Design review of the part built by this model. Coordinates are the model's own, in mm. A direction names the side the tool comes from. Round coordinates to 2 decimals unless told otherwise and drop trailing zeros. Loops run counter-clockwise (first coordinate to the right, second up) from the corner with the lowest first, then second, coordinate; pieces in that order, holes last. Notation, with made-up numbers: (-32.5, 52) - (25.5, 52) arc R6 cw to (25.5, 57) - close; hole circle Ø10 at (33, 34.5). An arc over 180 degrees is marked (long way). Return JSON: item names as keys, results as strings. Group by question number.
(1) We need section A-A, the plane x = 0. Write out the cut boundary in (y, z).
(2) The part is to be moulded in two halves that separate along Z. For faces 4 (the flat face through (50, 22, -32.75)), 5 (the flat face through (-50, 22, -32.75)), 6 (the flat face through (50, 40, -39)), 7 (the cylindrical face through (-34.471, -2.465, -83.137)), say which applies: pulls with the +Z half, pulls with the -Z half, needs draft (parallel to the pull), parting line crosses it, or undercut.
(3) We need section B-B, the plane z = -12.5. Write out the cut boundary in (x, y).
(4) For faces 1 (the flat face through (-37, 175, 35)), 2 (the flat face through (53.17, 22, -38)), 3 (the cylindrical face through (47.69, 177.54, 15.02)), list the 3-axis set-ups (+Z, -Z, +X, -X, +Y, -Y) from which the entire face can be reached by the end or side of a thin tool; tool diameter is ignored.
(5) Wall thickness on L1, parallel to Y at x = -12, z = -76.5; L2, parallel to Z at x = 0, y = 177.4; L3, parallel to Z at x = 0, y = 139.5: over which ranges is each line inside the solid? List them lowest first. Write a range as [from, to].
(6) Clearance check with flat-ended pins moving along their axes: pin 1 (2 mm diameter, centred on x = -50.5, y = 23, fed in from -Z); pin 2 (8 mm diameter, centred on y = 132, z = -12, fed in from +X); pin 3 (3 mm diameter, centred on x = -48.5, y = 26.5, fed in from +Z). State where each tip first meets the part, or that it passes through.
(7) We need section C-C, the plane y = 43. Write out the cut boundary in (x, z), and give its area (4 significant figures).
from build123d import *
from build123d.topology import SkipClean

# Parameters (mm, degrees)
BOSS_EXTRU_1_DEPTH      = 5
BOSS_EXTRU_2_DEPTH      = 180
BOSS_EXTRU_3_DEPTH      = 5
ENL_V_MAT_EXTRU_1_DEPTH = 5
BOSS_EXTRU_4_DEPTH      = 40
BOSS_EXTRU_5_DEPTH      = 5
ESQUISSE8_R             = 90
BOSS_EXTRU_6_DEPTH      = 5
BOSS_EXTRU_7_DEPTH      = 5
BOSS_EXTRU_8_DEPTH      = 5
ESQUISSE12_W            = 6.5
ESQUISSE12_H            = 11.508229801
ESQUISSE12_H_2          = 11.51
BOSS_EXTRU_9_DEPTH      = 35


with BuildPart() as part:
    # Esquisse1 → Boss.-Extru.1 (new body)
    with BuildSketch(Plane(origin=(0, 0, 0), x_dir=(1, 0, 0), z_dir=(0, 1, 0))):
        with BuildLine():
            ThreePointArc((0, 77.5), (-54.800775542, 54.800775542), (-77.5, 0))
            Line((-77.5, 0), (0, 0))
            Line((0, 0), (77.5, 0))
            ThreePointArc((77.5, 0), (54.800775542, 54.800775542), (0, 77.5))
        make_face()
    extrude(amount=BOSS_EXTRU_1_DEPTH)

    # Esquisse2 → Boss.-Extru.2 (add)
    with BuildSketch(Plane.XZ):
        with BuildLine():
            Line((80, 0), (77.5, 0))
            ThreePointArc((77.5, 0), (0, -77.5), (-77.5, 0))
            Line((-77.5, 0), (-80, 0))
            ThreePointArc((-80, 0), (0, -80), (80, 0))
        make_face()
    extrude(amount=-BOSS_EXTRU_2_DEPTH)

    # Esquisse4 → Boss.-Extru.3 (add)
    with BuildSketch(Plane(origin=(0, 180, 0), x_dir=(1, 0, 0), z_dir=(0, 1, 0))):
        with BuildLine():
            Line((-77.5, 0), (77.5, 0))
            ThreePointArc((77.5, 0), (0, 77.5), (-77.5, 0))
        make_face()
    extrude(amount=-BOSS_EXTRU_3_DEPTH)

    # Esquisse5 → Enlèv. mat.-Extru.1 (cut)
    with BuildSketch(Plane(origin=(0, 180, 0), x_dir=(1, 0, 0), z_dir=(0, 1, 0))):
        with BuildLine():
            Line((-50, 0), (50, 0))
            ThreePointArc((50, 0), (0, 50), (-50, 0))
        make_face()
    extrude(amount=-ENL_V_MAT_EXTRU_1_DEPTH, mode=Mode.SUBTRACT)

    # Esquisse6 → Boss.-Extru.4 (add)
    with SkipClean():  # the faces are left unmerged after this step: merging them gives an invalid solid
        with BuildSketch(Plane(origin=(0, 0, 0), x_dir=(1, 0, 0), z_dir=(0, 1, 0))):
            with BuildLine():
                Line((80, 0), (77.5, 0))
                ThreePointArc((77.5, 0), (0, -77.5), (-77.5, 0))
                Line((-77.5, 0), (-80, 0))
                ThreePointArc((-80, 0), (0, -80), (80, 0))
            make_face()
        extrude(amount=BOSS_EXTRU_4_DEPTH)

    # Esquisse7 → Boss.-Extru.5 (add)
    with BuildSketch(Plane(origin=(0, 0, 0), x_dir=(1, 0, 0), z_dir=(0, 1, 0))):
        with BuildLine():
            Line((0, 0), (-77.5, 0))
            ThreePointArc((-77.5, 0), (0, -77.5), (77.5, 0))
            Line((77.5, 0), (0, 0))
        make_face()
    extrude(amount=BOSS_EXTRU_5_DEPTH)

    # Esquisse8 → Boss.-Extru.6 (add)
    with BuildSketch(Plane.XZ):
        with Locations(Location((0, 0, 0), (0, 0, 270))):
            Circle(ESQUISSE8_R)
    extrude(amount=BOSS_EXTRU_6_DEPTH)



with BuildPart() as body_2:
    # Esquisse9 → Boss.-Extru.7 (new body)
    with BuildSketch(Plane(origin=(0, 180, 0), x_dir=(1, 0, 0), z_dir=(0, 1, 0))):
        with BuildLine():
            Line((80, 0), (77.5, 0))
            ThreePointArc((77.5, 0), (0, -77.5), (-77.5, 0))
            Line((-77.5, 0), (-80, 0))
            ThreePointArc((-80, 0), (0, -80), (80, 0))
        make_face()
    extrude(amount=-BOSS_EXTRU_7_DEPTH)


with BuildPart() as part_1:
    add(part.part)

    add(body_2.part)  # Boss.-Extru.8 merges body 2
    # Esquisse10 → Boss.-Extru.8 (add)
    with BuildSketch(Plane(origin=(0, 180, 0), x_dir=(1, 0, 0), z_dir=(0, 1, 0))):
        with BuildLine():
            ThreePointArc((-77.5, 0), (0, -77.5), (77.5, 0))
            Line((77.5, 0), (50, 0))
            ThreePointArc((50, 0), (0, -50), (-50, 0))
            Line((-50, 0), (-77.5, 0))
        make_face()
    extrude(amount=-BOSS_EXTRU_8_DEPTH)

    # Esquisse12 → Boss.-Extru.9 (add)
    with BuildSketch(Plane(origin=(0, 5, 0), x_dir=(1, 0, 0), z_dir=(0, 1, 0))):
        with Locations((-49.92, 38.5041149)):
            Rectangle(ESQUISSE12_W, ESQUISSE12_H)
        with Locations((49.92, 38.505)):
            Rectangle(ESQUISSE12_W, ESQUISSE12_H_2)
    extrude(amount=BOSS_EXTRU_9_DEPTH)


solid = part_1.part
Solutions:
{
 "1": {"outline": "(-5, -90) - (0, -90) - (0, -80) - (180, -80) - (180, -50) - (175, -50) - (175, -77.5) - (5, -77.5) - (5, 77.5) - (40, 77.5) - (40, 80) - (0, 80) - (0, 90) - (-5, 90) - close; (175, 50) - (180, 50) - (180, 80) - (175, 80) - close"},
 "2": {"face 4": "undercut", "face 5": "undercut", "face 6": "needs draft", "face 7": "parting line crosses it"},
 "3": {"outline": "(-89.13, -5) - (89.13, -5) - (89.13, 0) - (79.02, 0) - (79.02, 180) - (48.41, 180) - (48.41, 175) - (76.49, 175) - (76.49, 5) - (-76.49, 5) - (-76.49, 175) - (-48.41, 175) - (-48.41, 180) - (-79.02, 180) - (-79.02, 0) - (-89.13, 0) - close"},
 "4": {"face 1": "+Z", "face 2": "none", "face 3": "+Y"},
 "5": {"L1": "[-5, 5], [175, 180]", "L2": "[-80, -50], [50, 80]", "L3": "[-80, -77.5]"},
 "6": {"pin 1": "z = -62.85", "pin 2": "x = 79.6", "pin 3": "z = 64.74"},
 "7": {"outline": "(-80, 0) arc R80 ccw to (80, 0) - (77.5, 0) arc R77.5 cw to (-77.5, 0) - close", "area": "618.5 mm^2"}
}
